Check sheet for the modelled part. Datum: model origin and axes. Units: mm. Face numbers are marked on the shaded views. A direction names the side the tool comes from. Coordinates: 2 decimals unless noted, no trailing zeros. Write each loop counter-clockwise with the first axis right and the second up, starting at its lowest first coordinate (ties: lowest second). Pieces come first, ordered by that corner, then holes. Notation, with made-up numbers: (62, -37.75) -> (66, -37.75) arc R13 ccw to (66, -16.75) -> close; hole circle Ø11 at (33.25, 14). An arc over 180 degrees is marked (long way). One line per item, written item: value. Start each with the question number.
1) Sectioned sample at A-A on x = 203. Enter the section's corners in (y, z) (3 decimals).
2) Sectioned sample at B-B on y = 55. Enter the section's corners in (x, z), plus the area to 3 significant figures.
3) Draft check along Y on the marked faces 1, 2 and 3. Enter one of: +Y half, -Y half, draft (parallel to the pull), parting line (faces both ways), or undercut.
4) Sectioned sample at C-C on z = -57. Enter the section's corners in (x, y), plus the area to 3 significant figures.
5) Scan lines: line 1 along Y through (x, z) = (306.5, 31); line 2 along Z through (x, y) = (338.5, 23.5). Record each from-to range of solid material in increasing order. Write a range as [from, to].
6) Sectioned sample at D-D on x = 72.5. Enter the section's corners in (y, z) (3 decimals), plus the area to 3 significant figures.
7) Set-up check for the marked faces 4 and 5: record each of +Z, -Z, +X, -X, +Y, -Y from which the full face is reachable in a straight line by a thin tool's end or side.
```python
from build123d import *

# Parameters (mm, degrees)
F1_DEPTH = 466.973412
F3_DEPTH = 152.401
F4_R     = 5.08


with BuildPart() as f1:
    # F0 (on Right) → F1 (new body)
    with BuildSketch(Plane.YZ):
        with BuildLine():
            Line((73.025, 76.2), (-76.2, 76.2))
            Line((-76.2, 76.2), (-76.2, -76.2))
            Line((-76.2, -76.2), (73.025, -76.2))
            ThreePointArc((73.025, -76.2), (75.270064, -75.270064), (76.2, -73.025))
            Line((76.2, -73.025), (76.2, 73.025))
            ThreePointArc((76.2, 73.025), (75.270064, 75.270064), (73.025, 76.2))
        make_face()
        with BuildLine():
            Line((-69.850001, -66.674999), (-69.850001, 66.675001))
            ThreePointArc((-69.850001, 66.675001), (-68.920065, 68.920065), (-66.675001, 69.850001))
            Line((-66.675001, 69.850001), (66.675001, 69.850001))
            ThreePointArc((66.675001, 69.850001), (68.920065, 68.920065), (69.850001, 66.675001))
            Line((69.850001, 66.675001), (69.850001, -66.674999))
            ThreePointArc((69.850001, -66.674999), (68.920065, -68.920063), (66.675001, -69.849999))
            Line((66.675001, -69.849999), (-66.675001, -69.849999))
            ThreePointArc((-66.675001, -69.849999), (-68.920065, -68.920063), (-69.850001, -66.674999))
        make_face(mode=Mode.SUBTRACT)
    extrude(amount=F1_DEPTH)

    # F2 (on face) → F3 (cut, through all)
    with BuildSketch(Plane.XZ.offset(76.2)):
        Polygon((0, 76.2), (0, -76.2), (152.4, 76.2), align=None)
        Polygon((314.573412, 76.2), (466.973412, -76.2), (466.973412, 76.2), align=None)
    extrude(amount=-F3_DEPTH, mode=Mode.SUBTRACT)

    # F4
    f4_edges = [f1.edges().sort_by_distance(p)[0] for p in [
        (233.486706, -76.2, 76.2),
        (233.486706, -76.2, -76.2),
    ]]
    fillet(f4_edges, radius=F4_R)


solid = f1.part
```
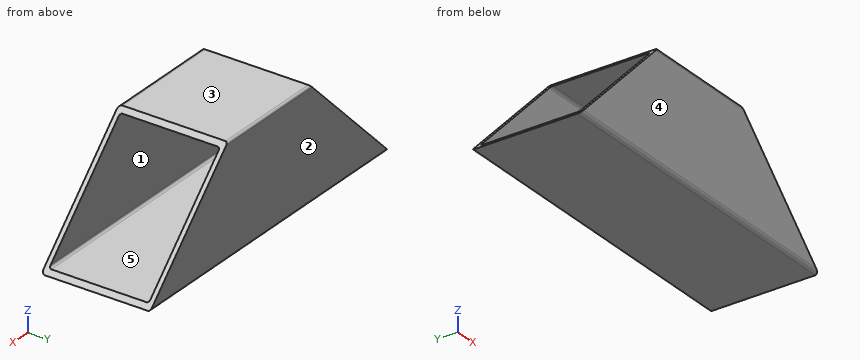
Answers:
1. outline: (-76.2, -71.12) arc R5.08 ccw to (-71.12, -76.2) -> (73.025, -76.2) arc R3.175 ccw to (76.2, -73.025) -> (76.2, 73.025) arc R3.175 ccw to (73.025, 76.2) -> (-71.12, 76.2) arc R5.08 ccw to (-76.2, 71.12) -> close; hole (-69.85, -66.675) arc R3.175 ccw to (-66.675, -69.85) -> (66.675, -69.85) arc R3.175 ccw to (69.85, -66.675) -> (69.85, 66.675) arc R3.175 ccw to (66.675, 69.85) -> (-66.675, 69.85) arc R3.175 ccw to (-69.85, 66.675) -> close
2. outline: (0, -76.2) -> (466.97, -76.2) -> (460.62, -69.85) -> (6.35, -69.85) -> close; (146.05, 69.85) -> (320.92, 69.85) -> (314.57, 76.2) -> (152.4, 76.2) -> close
2. area: 4,000 mm2
3. face 1: undercut
3. face 2: +Y half
3. face 3: draft
4. outline: (19.2, -76.2) -> (447.77, -76.2) -> (447.77, -69.85) -> (19.2, -69.85) -> close; (19.2, 69.85) -> (447.77, 69.85) -> (447.77, 76.2) -> (19.2, 76.2) -> close
4. area: 5,440 mm2
5. line 1: y = [-76.2, -69.85], [69.85, 76.2]
5. line 2: z = [-76.2, -69.85]
6. outline: (-76.2, -71.12) arc R5.08 ccw to (-71.12, -76.2) -> (73.025, -76.2) arc R3.175 ccw to (76.2, -73.025) -> (76.2, -3.7) -> (69.85, -3.7) -> (69.85, -66.675) arc R3.175 cw to (66.675, -69.85) -> (-66.675, -69.85) arc R3.175 cw to (-69.85, -66.675) -> (-69.85, -3.7) -> (-76.2, -3.7) -> close
6. area: 1,800 mm2
7. face 4: +Z, -Z, +X, -X, -Y
7. face 5: +X, -X
